Work out the finished part from the listing and answer in its coordinate system (mm). A direction names the side the tool comes from. Coordinates: 2 decimals unless noted, no trailing zeros. Loops run counter-clockwise (first coordinate to the right, second up) from the corner with the lowest first, then second, coordinate; pieces in that order, holes last. Notation, with made-up numbers: (52.5, -22) -> (102.5, -22) arc R20 cw to (102.5, 14) -> close; hole circle Ø4 at (-13.75, 43.5). An arc over 180 degrees is marked (long way). Use a Markdown table: item, result.
from build123d import *

# Parameters (mm, degrees)
BOSS_EXTRUDE1_DEPTH = 40
SKETCH2_R           = 5
BOSS_EXTRUDE2_DEPTH = 50


with BuildPart() as part:
    # Sketch1 → Boss-Extrude1 (new body)
    with BuildSketch(Plane.XY):
        Polygon((0, 10), (0, 35), (0, 45), (-25, 45), (-25, 35), (-10, 35), (-10, 10), (-25, 10), (-25, 0), (0, 0), align=None)
    extrude(amount=BOSS_EXTRUDE1_DEPTH)

    # Sketch2 → Boss-Extrude2 (add)
    with BuildSketch(Plane(origin=(0, 0, 0), x_dir=(0, 0, -1), z_dir=(1, 0, 0))):
        with Locations((-20, 22.5)):
            Circle(SKETCH2_R)
    extrude(amount=BOSS_EXTRUDE2_DEPTH)


solid = part.part
Q1. For faces 4 (the cylindrical face through (24.65, 17.62, 21.08)), 5 (the flat face through (-17, 10, 20)), 6 (the flat face through (-25, 5, 20)), determine the directions among +Z, -Z, +X, -X, +Y, -Y from which every point of the face is accessible in a straight line to the end or side of a thin tool.
Solved:
| item | result |
|---|---|
| face 4 | +X |
| face 5 | +Z, -Z, -X |
| face 6 | +Z, -Z, -X, +Y, -Y |
Q2. Determine the mould class of faces 1 (the flat face through (-18, 35, 20)), 2 (the flat face through (-25, 40, 20)), 3 (the flat face through (-13, 0, 20)) for opening direction Y: pulls with the +Y half, pulls with the -Y half, needs draft (parallel to the pull), parting line crosses it, or undercut.
Solved:
| item | result |
|---|---|
| face 1 | undercut |
| face 2 | needs draft |
| face 3 | pulls with the -Y half |
Q3. Section B-B on y = 22.5 is taken. Determine the outline of the cut face in (x, z).
Solved:
| item | result |
|---|---|
| outline | (-10, 0) -> (0, 0) -> (0, 15) -> (50, 15) -> (50, 25) -> (0, 25) -> (0, 40) -> (-10, 40) -> close |
Q4. Given pin 1 Ø12 at (x, y) = (21.5, 15) entering from -Z; pin 2 Ø12 at (y, z) = (22, 31) entering from -X; pin 3 Ø8 at (x, y) = (15.5, 16.5) entering from -Z, each flat-ended and moving along its own axis, determine where each tip first touches the part or whether it passes through.
Solved:
| item | result |
|---|---|
| pin 1 | z = 15.23 |
| pin 2 | x = -10 |
| pin 3 | z = 15.42 |
Q5. Section D-D on z = 9 is taken. Determine the outline of the cut face in (x, y).
Solved:
| item | result |
|---|---|
| outline | (-25, 0) -> (0, 0) -> (0, 45) -> (-25, 45) -> (-25, 35) -> (-10, 35) -> (-10, 10) -> (-25, 10) -> close |
Q6. Consider line 1 (Y direction, x = -12.5, z = 13); line 2 (X direction, y = 17, z = 17); line 3 (X direction, y = 39, z = 14). Determine where each line is inside the solid, lowest interval first. Write a range as [from, to].
Solved:
| item | result |
|---|---|
| line 1 | [0, 10], [35, 45] |
| line 2 | [-10, 0] |
| line 3 | [-25, 0] |
Q7. Section A-A on z = 23 is taken. Determine the outline of the cut face in (x, y).
Solved:
| item | result |
|---|---|
| outline | (-25, 0) -> (0, 0) -> (0, 18.5) -> (50, 18.5) -> (50, 26.5) -> (0, 26.5) -> (0, 45) -> (-25, 45) -> (-25, 35) -> (-10, 35) -> (-10, 10) -> (-25, 10) -> close |
Q8. Section C-C on x = 17 is taken. Determine the outline of the cut face in (y, z).
Solved:
| item | result |
|---|---|
| outline | circle Ø10 at (22.5, 20) |
